from build123d import *

# Parameters (mm, degrees)
EXTRUDE_THIN1_DEPTH = 19.05
CUT_EXTRUDE1_REACH  = 97.25
SKETCH2_R           = 6.35


with BuildPart() as part:
    # Sketch1 → Extrude-Thin1 (new body, symmetric)
    with BuildSketch(Plane(origin=(0, 0, 0), x_dir=(0, 0, -1), z_dir=(1, 0, 0))):
        with BuildLine():
            Line((-77.216478592, 27.494340102), (-45.335245167, 0.742808893))
            ThreePointArc((-45.335245167, 0.742808893), (-44.380308461, 0.191475929), (-43.294394506, 0))
            Line((-43.294394506, 0), (-3.175, 0))
            ThreePointArc((-3.175, 0), (-0.92993597, 0.92993597), (0, 3.175))
            Line((0, 3.175), (0, 79.375))
            ThreePointArc((0, 79.375), (-0.92993597, 81.62006403), (-3.175, 82.55))
            Line((-3.175, 82.55), (-57.15, 82.55))
            Line((-57.15, 82.55), (-57.15, 88.9))
            Line((-57.15, 88.9), (-3.175, 88.9))
            ThreePointArc((-3.175, 88.9), (3.560192091, 86.110192091), (6.35, 79.375))
            Line((6.35, 79.375), (6.35, 3.175))
            ThreePointArc((6.35, 3.175), (3.560192091, -3.560192091), (-3.175, -6.35))
            Line((-3.175, -6.35), (-43.294394506, -6.35))
            ThreePointArc((-43.294394506, -6.35), (-46.552136371, -5.775572213), (-49.416946488, -4.121573321))
            Line((-49.416946488, -4.121573321), (-81.298179914, 22.629957888))
            Line((-81.298179914, 22.629957888), (-77.216478592, 27.494340102))
        make_face()
    extrude(amount=EXTRUDE_THIN1_DEPTH, both=True)

    # Sketch2 → Cut-Extrude1 (cut, up to next)
    with BuildSketch(Plane(origin=(0, 88.9, 0), x_dir=(1, 0, 0), z_dir=(0, 1, 0)), mode=Mode.PRIVATE) as cut_extrude1_sk1:
        with Locations((0, -38.1)):
            Circle(SKETCH2_R)
    cut_extrude1_tool1 = extrude(cut_extrude1_sk1.sketch, amount=-CUT_EXTRUDE1_REACH, mode=Mode.PRIVATE) & part.part
    add(cut_extrude1_tool1.solids().sort_by_distance((0, 88.9, 38.1))[0], mode=Mode.SUBTRACT)


solid = part.part
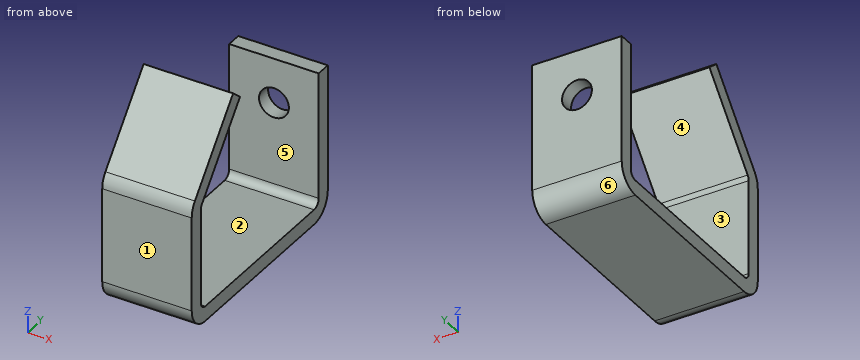
Here's how the part is built. I have some questions about the finished solid (model axes, mm). Face numbers are marked on the shaded views. A direction names the side the tool comes from. Round coordinates to 2 decimals unless told otherwise and drop trailing zeros. Loops run counter-clockwise (first coordinate to the right, second up) from the corner with the lowest first, then second, coordinate; pieces in that order, holes last. Notation, with made-up numbers: (-31, 66) - (7, 66) arc R28 cw to (7, 91) - close; hole circle Ø10 at (-4.75, 12.5). An arc over 180 degrees is marked (long way). One line per question, with ' | ' between items. Start each with the question number.
Q1. I want a section at D-D (x = 11). Write out the boundary of the cut face in (y, z) (3 decimals).
Q2. Please list where these lines run through material, in increasing order: line 1 (X direction, y = 87, z = 38.1); line 2 (Z direction, x = 0, y = 85.5); line 3 (Y direction, x = -11, z = 35). Write a range as [from, to].
Q3. Will these pins go through, and if not, where does the flat tip stop? pin 1 (1.5 mm diameter, centred on x = 14, z = 69, fed in from -Y); pin 2 (5 mm diameter, centred on x = -1.5, y = 87, fed in from +Z).
Q4. I want a section at C-C (z = 38.1). Write out the boundary of the cut face in (x, y), then the cut area to 3 significant figures.
Q5. For the marked faces 1 and 2, which set-ups out of +Z, -Z, +X, -X, +Y, -Y let a thin tool reach every point of the face, with its end or its side?
Q6. I want a section at B-B (x = 0). Write out the boundary of the cut face in (y, z) (3 decimals), then the cut area to 3 significant figures.
Q7. I want a section at A-A (z = 6.5). Write out the boundary of the cut face in (x, y), then the cut area to 3 significant figures.
Q8. We'd pull the mould along Z, two halves only. Please class the marked faces 3, 4, 5 and 6: +Z half, -Z half, draft (parallel to the pull), parting line (faces both ways), or undercut.
Response values:
1) outline: (-6.35, 3.175) arc R9.525 ccw to (3.175, -6.35) - (79.375, -6.35) arc R9.525 ccw to (88.9, 3.175) - (88.9, 57.15) - (82.55, 57.15) - (82.55, 3.175) arc R3.175 cw to (79.375, 0) - (3.175, 0) arc R3.175 cw to (0, 3.175) - (0, 43.294) arc R3.175 cw to (0.743, 45.335) - (27.494, 77.216) - (22.63, 81.298) - (-4.122, 49.417) arc R9.525 ccw to (-6.35, 43.294) - close
2) line 1: x = [-19.05, -6.35], [6.35, 19.05] | line 2: z = [-4.12, 31.75], [44.45, 57.15] | line 3: y = [-6.35, 0], [82.55, 88.9]
3) pin 1: stops at y = 11.68 | pin 2: stops at z = 57.15
4) outline: (-19.05, -6.35) - (19.05, -6.35) - (19.05, 0) - (-19.05, 0) - close; (-19.05, 82.55) - (-6.35, 82.55) - (-6.35, 88.9) - (-19.05, 88.9) - close; (6.35, 82.55) - (19.05, 82.55) - (19.05, 88.9) - (6.35, 88.9) - close | area: 403 mm²
5) face 1: +Z, -Z, +X, -X, -Y | face 2: +X, -X
6) outline: (-6.35, 3.175) arc R9.525 ccw to (3.175, -6.35) - (79.375, -6.35) arc R9.525 ccw to (88.9, 3.175) - (88.9, 31.75) - (82.55, 31.75) - (82.55, 3.175) arc R3.175 cw to (79.375, 0) - (3.175, 0) arc R3.175 cw to (0, 3.175) - (0, 43.294) arc R3.175 cw to (0.743, 45.335) - (27.494, 77.216) - (22.63, 81.298) - (-4.122, 49.417) arc R9.525 ccw to (-6.35, 43.294) - close; (82.55, 44.45) - (88.9, 44.45) - (88.9, 57.15) - (82.55, 57.15) - close | area: 1,420 mm²
7) outline: (-19.05, -6.35) - (19.05, -6.35) - (19.05, 0) - (-19.05, 0) - close; (-19.05, 82.55) - (19.05, 82.55) - (19.05, 88.9) - (-19.05, 88.9) - close | area: 484 mm²
8) face 3: undercut | face 4: undercut | face 5: draft | face 6: -Z half
